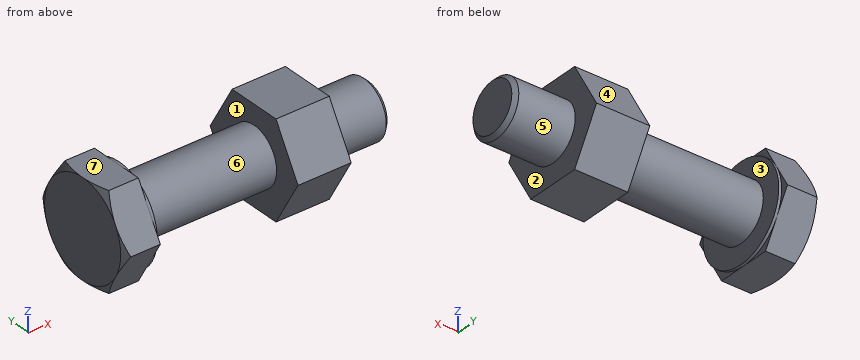
from build123d import *

# Parameters (mm, degrees)
BASEHEAD_DEPTH      = 10.32
SKETCH4_W           = 0.8
SKETCH4_H           = 12.088457268
BOSS_EXTRUDE2_DEPTH = 15


# Read off the part's stored shape, not the designer's step: HeadChamfer
with BuildPart() as part:
    # Sketch1 → BaseHead (new body)
    with BuildSketch(Plane(origin=(0, 0, 0), x_dir=(0, 0, -1), z_dir=(1, 0, 0))):
        Polygon((13.5, 7.794228634), (13.5, -7.794228634), (0, -15.588457268), (-13.5, -7.794228634), (-13.5, 7.794228634), (0, 15.588457268), align=None)
    extrude(amount=BASEHEAD_DEPTH)

    # HeadChamfer outline → HeadChamfer (revolve, cut)
    with BuildSketch(Plane.YX):
        Polygon((15.58845727, 1.205771367), (13.499999851, -8.6e-08), (15.58845727, -8.6e-08), align=None)
    revolve(axis=Axis((0, 0, 0), (1, 0, 0)), mode=Mode.SUBTRACT)

    # HeadChamfer 2 outline → HeadChamfer 2 (revolve)
    with BuildSketch(Plane.YX):
        Polygon((8, 10.32), (8, 79.2185), (6.8985, 80.32), (0, 80.32), (0, 10.32), align=None)
    revolve(axis=Axis((0, 0, 0), (1, 0, 0)))

    # Sketch4 → BearingFace (revolve, cut)
    with BuildSketch(Plane.XY, mode=Mode.PRIVATE) as bearingface_sk:
        with Locations((9.92, 19.544228634)):
            Rectangle(SKETCH4_W, SKETCH4_H)
    revolve(bearingface_sk.sketch.rotate(Axis((0, 0, 0), (1, 0, 0)), 90), axis=Axis((0, 0, 0), (1, 0, 0)), mode=Mode.SUBTRACT)

    # Sketch6 → Boss-Extrude2 (add)
    with BuildSketch(Plane(origin=(48.32, 0, 0), x_dir=(0, 0, -1), z_dir=(1, 0, 0))):
        Polygon((0, 15.588457268), (-13.5, 7.794228634), (-13.5, -7.794228634), (0, -15.588457268), (13.5, -7.794228634), (13.5, 7.794228634), align=None)
    extrude(amount=BOSS_EXTRUDE2_DEPTH)


solid = part.part
Geometry check sheet. Reference: the model listing, model coordinates, mm. Face numbers are marked on the shaded views. A direction names the side the tool comes from. Give positions to 0.01 mm unless a question says otherwise; leave off trailing zeros. Write each loop counter-clockwise with the first axis right and the second up, starting at its lowest first coordinate (ties: lowest second). Pieces come first, ordered by that corner, then holes.
1) Go/stop test with flat-tipped pins: pin 1 Ø3.5 at (y, z) = (-7, 10.5) entering from +X; pin 2 Ø12 at (x, y) = (20, 6) entering from +Z; pin 3 Ø2 at (x, z) = (48, 6.5) entering from +Y. Record where each tip stops, or that it passes through.
Values follow:
pin 1: stops at x = 63.32
pin 2: stops at z = 8
pin 3: stops at y = 12.38
2) Release check for a two-part mould opening along X. For the marked faces 1, 2, 3 and 4 record: released by +X, released by -X, zero draft, split by the parting line, or undercut.
Values follow:
face 1: undercut
face 2: released by +X
face 3: undercut
face 4: zero draft
3) Thickness scan on line 1 (X direction, y = -9, z = -2.5); line 2 (X direction, y = 13, z = -3.75); line 3 (Y direction, x = 57, z = 5.75). Record the ranges inside material, lowest first.
Values follow:
line 1: x = 0 to 10.32, 48.32 to 63.32
line 2: x = 0.02 to 9.52, 48.32 to 63.32
line 3: y = -12.27 to 12.27
4) Cross-section at A-A (x = 52). Record the boundary of the cut face in (y, z), plus the area to 3 significant figures.
Values follow:
outline: (-15.59, 0) - (-7.79, -13.5) - (7.79, -13.5) - (15.59, 0) - (7.79, 13.5) - (-7.79, 13.5) - close
area: 631 mm2
5) Cross-section at B-B (x = 71). Record the boundary of the cut face in (y, z).
Values follow:
outline: circle Ø16 at (0, 0)
6) Set-up check for the marked faces 5, 6 and 7: record each of +Z, -Z, +X, -X, +Y, -Y from which the full face is reachable in a straight line by a thin tool's end or side.
Values follow:
face 5: +X
face 6: none
face 7: +Z, +X, -X, +Y, -Y
